from build123d import *

# Parameters (mm, degrees)
F0_W     = 250
F0_H     = 750
F1_DEPTH = 500
F2_R     = 2
F3_DEPTH = 25
F4_R     = 2
F5_DEPTH = 25


with BuildPart() as f1:
    # F0 (on Top) → F1 (new body)
    with BuildSketch(Plane.XY):
        with Locations((-125, -375)):
            Rectangle(F0_W, F0_H)
        Polygon((-250, 0), (0, 0), (750, 0), (750, 250), (-250, 250), align=None)
    extrude(amount=F1_DEPTH)

    # F2 (on face) → F3 (cut)
    with BuildSketch(Plane.YZ):
        with Locations((-105, 300)):
            Circle(F2_R)
    extrude(amount=-F3_DEPTH, mode=Mode.SUBTRACT)

    # F4 (on face) → F5 (cut)
    with BuildSketch(Plane.XZ):
        with Locations((105, 300)):
            Circle(F4_R)
    extrude(amount=-F5_DEPTH, mode=Mode.SUBTRACT)


solid = f1.part
Here's how the part is built. I have some questions about the finished solid (model axes, mm). A direction names the side the tool comes from. Give positions to 0.01 mm unless a question says otherwise; leave off trailing zeros. Loops run counter-clockwise (first coordinate to the right, second up) from the corner with the lowest first, then second, coordinate; pieces in that order, holes last. Notation, with made-up numbers: (11, -29.5) -> (20, -29.5) arc R19 ccw to (20, 4.5) -> close; hole circle Ø11 at (77.25, 44.25). An arc over 180 degrees is marked (long way). Answer as a JSON object with one key per item and string values. Group by question number.
Item 1: Imagine slicing it at C-C on y = -165.5. Write out the boundary of the cut face in (x, z), then the cut area to 3 significant figures.
Item 2: Imagine slicing it at B-B on x = 347. Write out the boundary of the cut face in (y, z).
Item 3: Imagine slicing it at A-A on z = 359.5. Write out the boundary of the cut face in (x, y), then the cut area to 4 significant figures.
Item 4: I need wall thicknesses on L1, parallel to X at y = 18.25, z = 300; L2, parallel to Z at x = -10.5, y = -105; L3, parallel to Y at x = -6, z = 300. Which ranges of each line are inside material? Lowest first, please.
Item 5: On a 3-axis mill with a long thin cutter (end or side, diameter ignored), from which of +Z, -Z, +X, -X, +Y, -Y can I reach the whole of each face in a straight line? I mean faces 1 (the flat face through (370, 0, 246)), 2 (the flat face through (257, 250, 246)). Say none if no direction works.
Item 6: Will these pins go through, and if not, where does the flat tip stop? pin 1 (8 mm diameter, centred on y = -34.5, z = 368.5, fed in from +X); pin 2 (2 mm diameter, centred on y = -105, z = 300.5, fed in from +X); pin 3 (2 mm diameter, centred on x = 105.5, z = 301, fed in from -Y).
Answer list:
{
 "1": {"outline": "(-250, 0) -> (0, 0) -> (0, 500) -> (-250, 500) -> close", "area": "125,000 mm2"},
 "2": {"outline": "(0, 0) -> (250, 0) -> (250, 500) -> (0, 500) -> close"},
 "3": {"outline": "(-250, -750) -> (0, -750) -> (0, 0) -> (750, 0) -> (750, 250) -> (-250, 250) -> close", "area": "437,500 mm2"},
 "4": {"L1": "x = -250 to 103, 107 to 750", "L2": "z = 0 to 298, 302 to 500", "L3": "y = -750 to -107, -103 to 250"},
 "5": {"face 1": "+Z, -Z, +X, -Y", "face 2": "+Z, -Z, +X, -X, +Y"},
 "6": {"pin 1": "stops at x = 0", "pin 2": "stops at x = -25", "pin 3": "stops at y = 0"}
}
